Study the drawing (mm; zero at the part's minimum x, y, z) and answer. A direction names the side the tool comes from. Give positions to 0.01 mm unless a question says otherwise; leave off trailing zeros. Loops run counter-clockwise (first coordinate to the right, second up) from the corner with the lowest first, then second, coordinate; pieces in that order, holes last. Notation, with made-up numbers: M 73.5,-40 L 114.5,-40 A22 cw 114.5,-22 Z; hole C -9,-2 d4. An arc over 180 degrees is marked long. Use one line per item in the form item = value. Start each with the question number.
1. For the marked faces 1, 2, 3 and 4, determine the directions among +Z, -Z, +X, -X, +Y, -Y from which every point of the face is accessible in a straight line to the end or side of a thin tool.
2. A straight line is drawn through the part: line 1 (Y direction, x = 5.25, z = 2.3). Find the intervals that lie inside material, in ascending order. Write a range as from..to.
3. The part is cut by section A-A (z = 0.95). Write down the section's boundary in (x, y), and give its area (3 significant figures).
4. The part is cut by section B-B (x = 11.75). Write down the section's boundary in (y, z).
5. Each of these flat-tipped pins is pushed along its axis until it touches: pin 1 Ø1.5 at (x, z) = (14, 1.5) entering from -Y; pin 2 Ø0.8 at (y, z) = (69.5, 1) entering from -X. Where does it stop, or does it pass through?
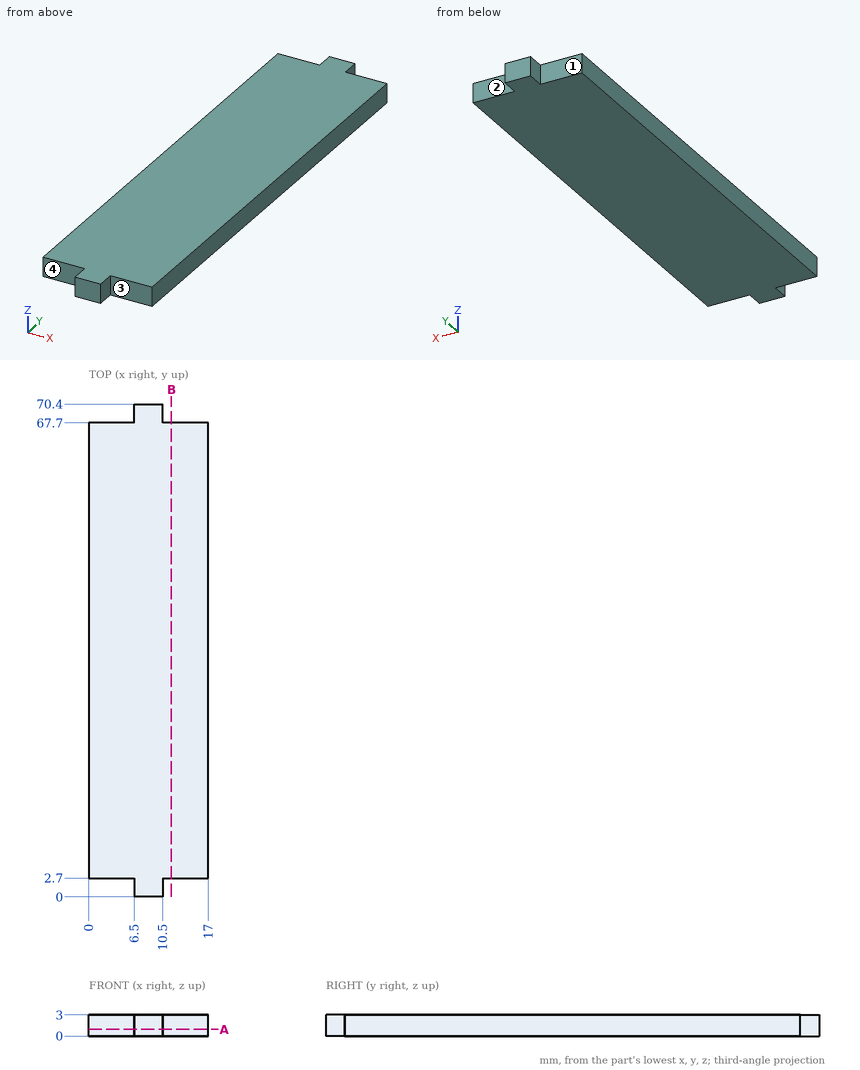
Derived:
q1.face_1 = +Z, -Z, -X, +Y
q1.face_2 = +Z, -Z, +X, +Y
q1.face_3 = +Z, -Z, +X, -Y
q1.face_4 = +Z, -Z, -X, -Y
q2.line_1 = 2.7..67.7
q3.outline = M 0,2.7 L 6.5,2.7 L 6.5,0 L 10.5,0 L 10.5,2.7 L 17,2.7 L 17,67.7 L 10.5,67.7 L 10.5,70.4 L 6.5,70.4 L 6.5,67.7 L 0,67.7 Z
q3.area = 1,130 mm2
q4.outline = M 2.7,0 L 67.7,0 L 67.7,3 L 2.7,3 Z
q5.pin_1 = 2.7
q5.pin_2 = 6.5
